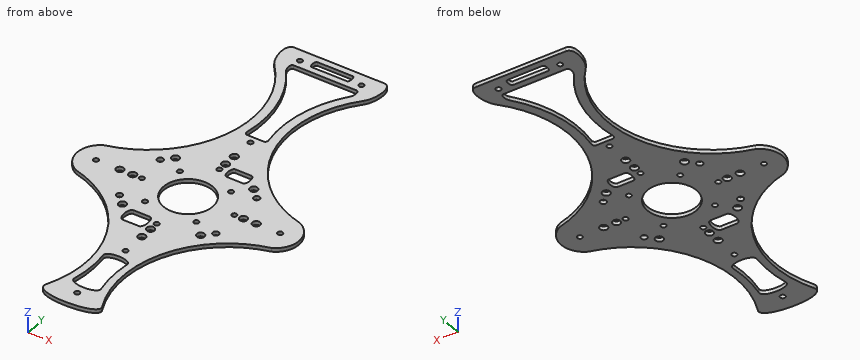
from build123d import *

# Parameters (mm, degrees)
MODEL_R         = 1
MODEL_R_2       = 1.5
MODEL_R_3       = 1.2
MODEL_R_4       = 9.672061212
EXTRUDE_1_DEPTH = 1.5


with BuildPart() as part:
    # Model → 凸台-拉伸1 (new body)
    with BuildSketch(Plane.XY):
        with BuildLine():
            Line((164.249855651, 187.088781669), (146.787217515, 187.088781669))
            Line((146.787217515, 187.088781669), (129.32457938, 187.088781669))
            add(Edge.make_bspline(
                [(129.32457938, 187.088781669), (125.461044671, 187.088781669), (126.746381631, 178.375641151), (129.32457938, 175.498177543)],
                knots=[0, 0, 0, 0, 11.590604126, 11.590604126, 11.590604126, 11.590604126], degree=3))
            ThreePointArc((129.32457938, 175.498177543), (139.773420004, 147.014985412), (127.780187237, 119.146851779))
            ThreePointArc((127.780187237, 119.146851779), (118.967335725, 112.447515783), (108.683438965, 108.350087077))
            ThreePointArc((108.683438965, 108.350087077), (103.514701902, 100.139821501), (108.683438965, 91.929555925))
            ThreePointArc((108.683438965, 91.929555925), (118.967335725, 87.832127219), (127.780187237, 81.132791223))
            ThreePointArc((127.780187237, 81.132791223), (139.177354468, 59.195873616), (135.89135677, 34.694322764))
            add(Edge.make_bspline(
                [(135.89135677, 34.694322764), (132.800282497, 28.120921276), (160.774152533, 29.120921276), (157.683078261, 34.694322764)],
                knots=[0, 0, 0, 0, 21.791721492, 21.791721492, 21.791721492, 21.791721492], degree=3))
            ThreePointArc((157.683078261, 34.694322764), (154.397080563, 59.195873616), (165.794247794, 81.132791223))
            ThreePointArc((165.794247794, 81.132791223), (174.607099306, 87.832127219), (184.890996066, 91.929555925))
            ThreePointArc((184.890996066, 91.929555925), (190.059733129, 100.139821501), (184.890996066, 108.350087077))
            ThreePointArc((184.890996066, 108.350087077), (174.607099306, 112.447515783), (165.794247794, 119.146851779))
            ThreePointArc((165.794247794, 119.146851779), (153.801015027, 147.014985412), (164.249855651, 175.498177543))
            add(Edge.make_bspline(
                [(164.249855651, 187.088781669), (168.11339036, 187.088781669), (166.8280534, 178.375641151), (164.249855651, 175.498177543)],
                knots=[0, 0, 0, 0, 11.590604126, 11.590604126, 11.590604126, 11.590604126], degree=3))
        make_face()
        with Locations((156.787217515, 110.139821501)):
            Circle(MODEL_R, mode=Mode.SUBTRACT)
        with Locations((136.787217515, 110.139821501)):
            Circle(MODEL_R, mode=Mode.SUBTRACT)
        with Locations((136.787217515, 90.139821501)):
            Circle(MODEL_R, mode=Mode.SUBTRACT)
        with Locations((156.787217515, 90.139821501)):
            Circle(MODEL_R, mode=Mode.SUBTRACT)
        with Locations((168.353974342, 100.139821501)):
            Circle(MODEL_R_2, mode=Mode.SUBTRACT)
        with Locations((146.787217515, 121.706578327)):
            Circle(MODEL_R_2, mode=Mode.SUBTRACT)
        with Locations((125.220460689, 100.139821501)):
            Circle(MODEL_R_2, mode=Mode.SUBTRACT)
        with Locations((146.787217515, 78.573064675)):
            Circle(MODEL_R_2, mode=Mode.SUBTRACT)
        with Locations((146.787217515, 126.706578327)):
            Circle(MODEL_R_2, mode=Mode.SUBTRACT)
        with Locations((120.220460689, 100.139821501)):
            Circle(MODEL_R_2, mode=Mode.SUBTRACT)
        with Locations((146.787217515, 73.573064675)):
            Circle(MODEL_R_2, mode=Mode.SUBTRACT)
        with Locations((173.353974342, 100.139821501)):
            Circle(MODEL_R_2, mode=Mode.SUBTRACT)
        with Locations((146.787217515, 118.171044401)):
            Circle(MODEL_R, mode=Mode.SUBTRACT)
        with Locations((128.755994615, 100.139821501)):
            Circle(MODEL_R, mode=Mode.SUBTRACT)
        with Locations((146.787217515, 82.108598601)):
            Circle(MODEL_R, mode=Mode.SUBTRACT)
        with Locations((164.818440415, 100.139821501)):
            Circle(MODEL_R, mode=Mode.SUBTRACT)
        with Locations((162.037217515, 115.389821501)):
            Circle(MODEL_R_2, mode=Mode.SUBTRACT)
        with Locations((131.537217515, 115.389821501)):
            Circle(MODEL_R_2, mode=Mode.SUBTRACT)
        with Locations((131.537217515, 84.889821501)):
            Circle(MODEL_R_2, mode=Mode.SUBTRACT)
        with Locations((162.037217515, 84.889821501)):
            Circle(MODEL_R_2, mode=Mode.SUBTRACT)
        with Locations((182.657217515, 100.139821501)):
            Circle(MODEL_R, mode=Mode.SUBTRACT)
        with Locations((146.787217515, 136.036864466)):
            Circle(MODEL_R, mode=Mode.SUBTRACT)
        with Locations((110.917217515, 100.139821501)):
            Circle(MODEL_R, mode=Mode.SUBTRACT)
        with Locations((146.787217515, 64.242778536)):
            Circle(MODEL_R, mode=Mode.SUBTRACT)
        with Locations((146.787217515, 36.419821501)):
            Circle(MODEL_R, mode=Mode.SUBTRACT)
        with Locations((158.787217515, 182.099821501)):
            Circle(MODEL_R, mode=Mode.SUBTRACT)
        with Locations((134.787217515, 182.099821501)):
            Circle(MODEL_R, mode=Mode.SUBTRACT)
        with Locations((128.00168361, 111.854287595)):
            Circle(MODEL_R_3, mode=Mode.SUBTRACT)
        with Locations((165.572751421, 111.854287595)):
            Circle(MODEL_R_3, mode=Mode.SUBTRACT)
        with Locations((128.00168361, 88.425355407)):
            Circle(MODEL_R_3, mode=Mode.SUBTRACT)
        with Locations((165.572751421, 88.425355407)):
            Circle(MODEL_R_3, mode=Mode.SUBTRACT)
        with Locations((146.787217515, 100.139821501)):
            Circle(MODEL_R_4, mode=Mode.SUBTRACT)
        with BuildLine():
            Line((159.067032454, 178.883153661), (146.787217515, 178.883153661))
            Line((146.787217515, 178.883153661), (134.507402577, 178.883153661))
            add(Edge.make_bspline(
                [(134.507402577, 178.883153661), (133.227688428, 178.883153661), (133.453062144, 176.072728685), (134.227836458, 175.05420374)],
                knots=[0, 0, 0, 0, 3.839142445, 3.839142445, 3.839142445, 3.839142445], degree=3))
            ThreePointArc((134.227836458, 175.05420374), (142.088179874, 158.46992126), (142.587324671, 140.123960438))
            add(Edge.make_bspline(
                [(142.587324671, 140.123960438), (142.493407811, 139.609308925), (142.9625841, 138.837088874), (143.485734707, 138.837088874)],
                knots=[0, 0, 0, 0, 1.56945182, 1.56945182, 1.56945182, 1.56945182], degree=3))
            Line((143.485734707, 138.837088874), (146.787217515, 138.837088874))
            Line((146.787217515, 138.837088874), (150.088700324, 138.837088874))
            add(Edge.make_bspline(
                [(150.98711036, 140.123960438), (151.08102722, 139.609308925), (150.611850931, 138.837088874), (150.088700324, 138.837088874)],
                knots=[0, 0, 0, 0, 1.56945182, 1.56945182, 1.56945182, 1.56945182], degree=3))
            ThreePointArc((150.98711036, 140.123960438), (151.486255157, 158.46992126), (159.346598573, 175.05420374))
            add(Edge.make_bspline(
                [(159.067032454, 178.883153661), (160.346746603, 178.883153661), (160.121372887, 176.072728685), (159.346598573, 175.05420374)],
                knots=[0, 0, 0, 0, 3.839142445, 3.839142445, 3.839142445, 3.839142445], degree=3))
        make_face(mode=Mode.SUBTRACT)
        with BuildLine():
            Line((151.053210178, 121.070269245), (157.209188782, 121.070269245))
            add(Edge.make_bspline(
                [(157.209188782, 121.070269245), (158.876955289, 121.070269245), (158.876955289, 116.066969722), (157.209188782, 116.066969722)],
                knots=[0, 0, 0, 0, 5.003299523, 5.003299523, 5.003299523, 5.003299523], degree=3))
            Line((157.209188782, 116.066969722), (151.053210178, 116.066969722))
            add(Edge.make_bspline(
                [(151.053210178, 121.070269245), (149.38544367, 121.070269245), (149.38544367, 116.066969722), (151.053210178, 116.066969722)],
                knots=[0, 0, 0, 0, 5.003299523, 5.003299523, 5.003299523, 5.003299523], degree=3))
        make_face(mode=Mode.SUBTRACT)
        with BuildLine():
            Line((136.47001729, 84.090392193), (142.625995894, 84.090392193))
            add(Edge.make_bspline(
                [(142.625995894, 84.090392193), (144.706817358, 84.090392193), (144.706817358, 77.847927799), (142.625995894, 77.847927799)],
                knots=[0, 0, 0, 0, 6.242464394, 6.242464394, 6.242464394, 6.242464394], degree=3))
            Line((142.625995894, 77.847927799), (136.47001729, 77.847927799))
            add(Edge.make_bspline(
                [(136.47001729, 84.090392193), (134.389195825, 84.090392193), (134.389195825, 77.847927799), (136.47001729, 77.847927799)],
                knots=[0, 0, 0, 0, 6.242464394, 6.242464394, 6.242464394, 6.242464394], degree=3))
        make_face(mode=Mode.SUBTRACT)
        with BuildLine():
            Line((139.974283877, 181.317718414), (153.600151154, 181.317718414))
            add(Edge.make_bspline(
                [(153.600151154, 184.631261375), (154.704665474, 184.631261375), (154.704665474, 181.317718414), (153.600151154, 181.317718414)],
                knots=[0, 0, 0, 0, 3.313542961, 3.313542961, 3.313542961, 3.313542961], degree=3))
            Line((153.600151154, 184.631261375), (139.974283877, 184.631261375))
            add(Edge.make_bspline(
                [(139.974283877, 184.631261375), (138.869769557, 184.631261375), (138.869769557, 181.317718414), (139.974283877, 181.317718414)],
                knots=[0, 0, 0, 0, 3.313542961, 3.313542961, 3.313542961, 3.313542961], degree=3))
        make_face(mode=Mode.SUBTRACT)
        with BuildLine():
            ThreePointArc((151.414191582, 58.179860404), (151.00262531, 50.30675556), (151.986875507, 42.484580784))
            add(Edge.make_bspline(
                [(141.587559524, 42.484580784), (140.851833579, 39.097117969), (152.722601452, 39.097117969), (151.986875507, 42.484580784)],
                knots=[0, 0, 0, 0, 10.399315983, 10.399315983, 10.399315983, 10.399315983], degree=3))
            ThreePointArc((141.587559524, 42.484580784), (142.57180972, 50.30675556), (142.160243449, 58.179860404))
            add(Edge.make_bspline(
                [(142.160243449, 58.179860404), (141.726972624, 61.233929522), (151.847462407, 61.233929522), (151.414191582, 58.179860404)],
                knots=[0, 0, 0, 0, 9.253948134, 9.253948134, 9.253948134, 9.253948134], degree=3))
        make_face(mode=Mode.SUBTRACT)
    extrude(amount=EXTRUDE_1_DEPTH)


solid = part.part
Here's how the part is built. I have some questions about the finished solid (model axes, mm). Round coordinates to 2 decimals unless told otherwise and drop trailing zeros. Loops run counter-clockwise (first coordinate to the right, second up) from the corner with the lowest first, then second, coordinate; pieces in that order, holes last.
1. If I drill on line 1 along Y through (x, z) = (145, 0.85); line 2 along Y through (x, z) = (148.5, 1.25); line 3 along X through (y, z) = (149, 1.45), over which ranges is the centre line in solid material (lowest first)?
Answer list:
line 1: y = 30.15 to 40.06, 60.33 to 90.63, 109.65 to 138.84, 178.88 to 181.32, 184.63 to 187.09
line 2: y = 30.21 to 40.05, 60.34 to 90.62, 109.66 to 138.84, 178.88 to 181.32, 184.63 to 187.09
line 3: x = 139.78 to 143.3, 150.27 to 153.79
2. If we section it at B-B on y = 151: Write out the boundary of the cut face in (x, z).
Answer list:
outline: (139.69, 0) - (143.22, 0) - (143.22, 1.5) - (139.69, 1.5) - close; (150.36, 0) - (153.89, 0) - (153.89, 1.5) - (150.36, 1.5) - close
3. If we section it at D-D on z = 0.25: Count the separate pieces of the cut face and the enclosed holes in it, plus the area to 3 significant figures.
Answer list:
separate pieces: 1
enclosed holes: 37
area: 3,870 mm2
4. If we section it at A-A on y = 46.5: Write out the boundary of the cut face in (x, z).
Answer list:
outline: (139.4, 0) - (142.27, 0) - (142.27, 1.5) - (139.4, 1.5) - close; (151.31, 0) - (154.18, 0) - (154.18, 1.5) - (151.31, 1.5) - close
5. For P1, Ø4, axis at x = 128, y = 111.85, coming from the -Z side; P2, Ø0.8, axis at x = 153, z = 1, coming from the -Y side, each with a flat end and sliding along its axis, tell me the tip position at first contact or that it passes through.
Answer list:
P1: stops at z = 0
P2: stops at y = 30.73
6. If we section it at C-C on x = 117: Write out the boundary of the cut face in (y, z).
Answer list:
outline: (88.87, 0) - (111.4, 0) - (111.4, 1.5) - (88.87, 1.5) - close
